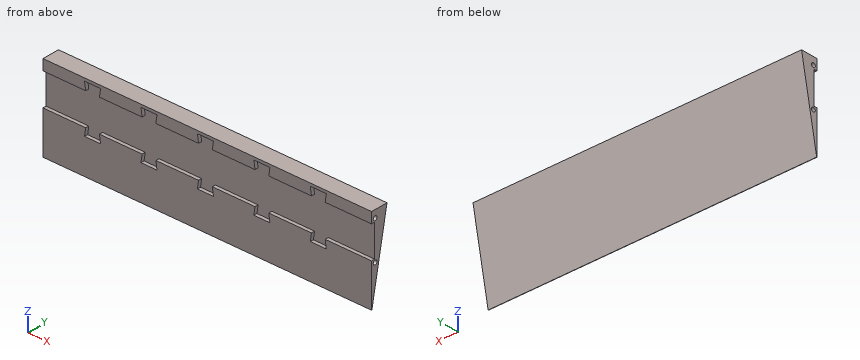
```python
from build123d import *

# Parameters (mm, degrees)
BOSS_EXTRUDE1_DEPTH = 195.58
SKETCH2_R           = 2.5527
CUT_EXTRUDE1_DEPTH  = 38.1
SKETCH3_W           = 38.1
SKETCH3_H           = 4.064
CUT_EXTRUDE2_DEPTH  = 405.649982083
CUT_EXTRUDE3_DEPTH  = 4.064


with BuildPart() as part:
    # Sketch1 → Boss-Extrude1 (new, symmetric)
    with BuildSketch(Plane(origin=(0, 0, 0), x_dir=(0, 0, -1), z_dir=(1, 0, 0))):
        Polygon((0, 0), (0, 20.32), (101.6, 0.4), (101.6, 0), align=None)
    extrude(amount=BOSS_EXTRUDE1_DEPTH, both=True)

    # Sketch2 → Cut-Extrude1 (cut)
    with BuildSketch(Plane(origin=(195.58, 0, 0), x_dir=(0, 0, -1), z_dir=(1, 0, 0))):
        with Locations((8.876362872, 4.7625)):
            Circle(SKETCH2_R)
        with Locations((54.596362872, 4.7625)):
            Circle(SKETCH2_R)
    cut_extrude1 = extrude(amount=-CUT_EXTRUDE1_DEPTH, mode=Mode.SUBTRACT)

    # Mirror3: Cut-Extrude1 across plane
    add(cut_extrude1.mirror(Plane(origin=(0, 0, 0), x_dir=(0, 0, 1), z_dir=(1, 0, 0))), mode=Mode.SUBTRACT)

    # Sketch3 → Cut-Extrude2 (cut, through all)
    with BuildSketch(Plane.ZY.offset(195.58)):
        with Locations((-31.75, 2.032)):
            Rectangle(SKETCH3_W, SKETCH3_H)
    extrude(amount=-CUT_EXTRUDE2_DEPTH, mode=Mode.SUBTRACT)

    # Sketch4 → Cut-Extrude3 (cut)
    with BuildSketch(Plane.XZ):
        Polygon((-144.78, -50.8), (-146.105623787, -60.232303355), (-144.78, -60.232303355), (-128.381247573, -60.232303355), (-127.055623787, -60.232303355), (-128.381247573, -50.8), align=None)
        Polygon((-77.581247573, -50.8), (-78.90687136, -60.232303355), (-77.581247573, -60.232303355), (-61.182495147, -60.232303355), (-59.85687136, -60.232303355), (-61.182495147, -50.8), align=None)
        Polygon((-10.382495147, -50.8), (-11.708118933, -60.232303355), (-10.382495147, -60.232303355), (6.01625728, -60.232303355), (7.341881067, -60.232303355), (6.01625728, -50.8), align=None)
        Polygon((56.81625728, -50.8), (55.490633493, -60.232303355), (56.81625728, -60.232303355), (73.215009707, -60.232303355), (74.540633493, -60.232303355), (73.215009707, -50.8), align=None)
        Polygon((124.015009707, -50.8), (122.68938592, -60.232303355), (124.015009707, -60.232303355), (140.413762134, -60.232303355), (141.73938592, -60.232303355), (140.413762134, -50.8), align=None)
        Polygon((124.015009707, -12.7), (140.413762134, -12.7), (141.73938592, -3.267696645), (140.413762134, -3.267696645), (124.015009707, -3.267696645), (122.68938592, -3.267696645), align=None)
        Polygon((56.81625728, -12.7), (73.215009707, -12.7), (74.540633493, -3.267696645), (73.215009707, -3.267696645), (56.81625728, -3.267696645), (55.490633493, -3.267696645), align=None)
        Polygon((-10.382495147, -12.7), (6.01625728, -12.7), (7.341881067, -3.267696645), (6.01625728, -3.267696645), (-10.382495147, -3.267696645), (-11.708118933, -3.267696645), align=None)
        Polygon((-77.581247573, -12.7), (-61.182495147, -12.7), (-59.85687136, -3.267696645), (-61.182495147, -3.267696645), (-77.581247573, -3.267696645), (-78.90687136, -3.267696645), align=None)
        Polygon((-144.78, -12.7), (-128.381247573, -12.7), (-127.055623787, -3.267696645), (-128.381247573, -3.267696645), (-144.78, -3.267696645), (-146.105623787, -3.267696645), align=None)
    extrude(amount=-CUT_EXTRUDE3_DEPTH, mode=Mode.SUBTRACT)


solid = part.part
```
Could you check a few things on this model? Use its own coordinates, in mm. Round coordinates to 2 decimals unless told otherwise and drop trailing zeros. Write each loop counter-clockwise with the first axis right and the second up, starting at its lowest first coordinate (ties: lowest second). Pieces come first, ordered by that corner, then holes.
(1) For pin 1 (4 mm diameter, centred on y = 4.76, z = -8.88, fed in from +X); pin 2 (4.5 mm diameter, centred on y = 4.76, z = -54.6, fed in from -X); pin 3 (10 mm diameter, centred on x = 60.5, z = -39, fed in from +Y), each with a flat end and sliding along its axis, tell me the tip position at first contact or that it passes through.
Findings below:
pin 1: stops at x = 157.48
pin 2: stops at x = -157.48
pin 3: stops at y = 13.65
(2) Suppose I cut it at C-C on y = 12.5. Write out the boundary of the cut face in (x, z), and give its area (3 significant figures).
Findings below:
outline: (-195.58, -39.89) - (195.58, -39.89) - (195.58, 0) - (-195.58, 0) - close
area: 15,600 mm2
(3) Suppose I cut it at B-B on z = -63.5. Write out the boundary of the cut face in (x, y).
Findings below:
outline: (-195.58, 0) - (195.58, 0) - (195.58, 7.87) - (-195.58, 7.87) - close
(4) Suppose I cut it at A-A on x = -72.5. Write out the boundary of the cut face in (y, z).
Findings below:
outline: (0, -101.6) - (0.4, -101.6) - (20.32, 0) - (0, 0) - (0, -3.27) - (4.06, -3.27) - (4.06, -60.23) - (0, -60.23) - close
(5) If I drill on probe 1 along Y at (x, z) = (91, -73); probe 2 along Y at (x, z) = (-144, -63), over which ranges is the centre line in solid material (lowest first)?
Findings below:
probe 1: y = 0 to 6.01
probe 2: y = 0 to 7.97
